CAD build for the part. Positions are in the model's coordinates, mm. A direction names the side the tool comes from. Round coordinates to 2 decimals unless told otherwise and drop trailing zeros. Order: outer loops, then holes, each group sorted by start corner. A loop starts at its lowest first (then second) coordinate and runs counter-clockwise, first axis right, second up.
Autodesk Inventor part; units mm, degrees
ref_plane "YZ Plane" through (0, 0, 0) normal (1, 0, 0) x (0, 1, 0)
ref_plane "XZ Plane" through (0, 0, 0) normal (0, 1, 0) x (-1, 0, 0)
ref_plane "XY Plane" through (0, 0, 0) normal (0, 0, 1) x (1, 0, 0)
sketch "Sketch1" plane through (0, 0, 0) normal (0, 1, 0) x (-1, 0, 0)
  line L0 (0, 0) -> (170, 0)
  line L1 (170, 0) -> (170, -132.9)
  line L2 (0, -132.9) -> (0, 0)
  line L3 (170, -132.9) -> (95, -132.9)
  line L4 (75, -132.9) -> (0, -132.9)
  line L5 (95, -132.9) -> (95, -127.9)
  line L6 (95, -127.9) -> (75, -127.9)
  line L7 (75, -127.9) -> (75, -132.9)
  dimension "d0" = 132.9
  dimension "d22" = 170
  dimension "d23" = 75
  dimension "d24" = 75
  dimension "d41" = 5
  dimension "d42" = 5
  dimension "d43" = 75
  dimension "d44" = 20
extrude "Extrusion1" add sketch "Sketch1" along normal blind 4.7625
sketch "Sketch2" plane through (0, 4.7625, 0) normal (0, 1, 0) x (1, 0, 0)
  line L0 (-170, 0) -> (0, 0)
  line L1 (0, 132.9) -> (-170, 132.9)
  line L2 (-170, 0) -> (-170, 132.9)
  line L3 (-170, 132.9) -> (-165.2375, 132.9)
  line L4 (-165.2375, 132.9) -> (-165.2375, 0)
  line L5 (-170, 0) -> (-165.2375, 0)
  line L6 (0, 0) -> (-4.7625, 0)
  line L7 (-4.7625, 0) -> (-4.7625, 132.9)
  line L8 (-4.7625, 132.9) -> (0, 132.9)
  line L9 (0, 0) -> (0, 132.9)
  line L10 (0, 132.9) -> (0, 0)
  dimension "d4" = 4.7625
  dimension "d5" = 4.7625
extrude "Extrusion2" add sketch "Sketch2" along normal blind 85.2375 contours L7 L1 L9 L0
sketch "Sketch3" plane through (0, 4.7625, 0) normal (0, 1, 0) x (1, 0, 0)
  point P0 (0, 0)
sketch "Sketch4" plane through (-170, 0, -132.9) normal (-1, 0, 0) x (0, 0, 1)
  line L0 (132.9, 4.7625) -> (217.7528, 89.6153)
  line L1 (0, 4.7625) -> (132.9, 4.7625)
  line L2 (132.9, 0) -> (132.9, 4.7625)
  line L3 (0, 0) -> (132.9, 0)
  line L4 (132.9, 0) -> (220.1341, 87.2341)
  line L5 (220.1341, 87.2341) -> (217.7528, 89.6153)
  line L6 (132.9, 4.7625) -> (132.9, 0)
  dimension "d8" = 120
  dimension "d9" = 45
sketch "Sketch5" plane through (0, 0, 0) normal (1, 0, 0) x (0, 0, -1)
  line L0 (0, 0) -> (0, 90)
  line L1 (0, 90) -> (-90, 90)
  line L2 (132.9, 0) -> (0, 0)
  line L3 (-90, 90) -> (0, 0)
  line L4 (0, 0) -> (0, 90)
  dimension "d11" = 45
extrude "Extrusion3" add sketch "Sketch5" against normal blind 105.2375
sketch "Sketch6" plane through (-105.2375, 0, 0) normal (-1, 0, 0) x (0, 0, 1)
  line L0 (0, 0) -> (0, 4.7625)
  line L1 (0, 4.7625) -> (0, 90)
  line L2 (-132.9, 90) -> (90, 90)
  line L3 (0, 90) -> (85.2375, 90)
  line L4 (85.2375, 90) -> (0, 4.7625)
  line L5 (0, 0) -> (90, 90)
extrude "Extrusion4" cut sketch "Sketch6" against normal blind 100.475 contours L1 L2 L4
sketch "Sketch7" plane through (-105.2375, 0, 0) normal (-1, 0, 0) x (0, 0, 1)
  line L0 (0, 4.7625) -> (0, 0)
  line L1 (0, 0) -> (90, 90)
  line L2 (85.2375, 90) -> (0, 4.7625)
  line L3 (90, 90) -> (85.2375, 90)
  line L4 (85.2375, 90) -> (0, 4.7625)
extrude "Extrusion5" add sketch "Sketch7" along normal blind 64.75
extrude "Extrusion6" add sketch "Sketch2" along normal blind 85.2375 contours L2 L1 L4 L0
sketch "Sketch8" plane through (-170, 0, -132.9) normal (-1, 0, 0) x (0, 0, 1)
  line L0 (0, 90) -> (222.9, 90)
  line L1 (132.9, 90) -> (218.1375, 90)
  line L2 (218.1375, 90) -> (132.9, 4.7625)
  line L3 (218.1375, 90) -> (132.9, 4.7625)
  line L4 (132.9, 4.7625) -> (132.9, 90)
  point P0 (132.9, 0)
extrude "Extrusion7" add sketch "Sketch8" against normal blind 4.7625
sketch "Sketch9" plane through (0, 0, -132.9) normal (1, 0, 0) x (0, 0, -1)
  line L0 (0, 0) -> (0, 90)
  line L1 (-5, 55) -> (0, 55)
  line L2 (0, 55) -> (0, 35)
  line L3 (0, 35) -> (-5, 35)
  line L4 (-5, 35) -> (-5, 55)
  line L5 (0, 90) -> (-222.9, 90)
  line L6 (0, 0) -> (-132.9, 0)
  dimension "d28" = 5
  dimension "d29" = 20
  dimension "d30" = 35
  dimension "d31" = 35
extrude "Extrusion8" cut sketch "Sketch9" against normal blind 4.7625
sketch "Sketch10" plane through (-170, 0, -132.9) normal (-1, 0, 0) x (0, 0, 1)
  line L0 (0, 0) -> (0, 90)
  line L1 (0, 55) -> (5, 55)
  line L2 (5, 55) -> (5, 35)
  line L3 (5, 35) -> (0, 35)
  line L4 (0, 35) -> (0, 55)
  line L5 (0, 90) -> (218.1375, 90)
  line L6 (132.9, 0) -> (0, 0)
  dimension "d34" = 20
  dimension "d35" = 5
  dimension "d36" = 35
  dimension "d37" = 35
extrude "Extrusion9" cut sketch "Sketch10" against normal blind 4.7625
fillet "Fillet1" radius 1 4 edges at (-167.6188, 55, -127.9) (-167.6188, 35, -127.9) (-2.3813, 35, -127.9) (-2.3813, 55, -127.9)
properties part number "OpticalDeviceMirrorPart"
1. Tool access for faces 5 (the face through (-75, 2, -130)), 6 (the face through (-84, 4.762, -66)), 7 (the face through (-168, 45, -127.9)): list every direction of +Z, -Z, +X, -X, +Y, -Y with a clear straight run to the whole face (end or side of a thin tool).
2. Pin check, flat tips, straight feed: P1, Ø1.4, axis at x = -86, y = 2, coming from the -Z side; P2, Ø6, axis at x = -29.5, y = 15, coming from the -Z side; P3, Ø1.5, axis at x = -61.5, y = 15, coming from the -Z side. Stop position of each tip, or through.
3. Cut at D-D, the plane z = -89. Write the cut outline in (x, y), and give its area (3 significant figures).
4. Cut at C-C, the plane x = -39. Write the cut outline in (y, z), and give its area (3 significant figures).
5. Drill centre lines: line 1 (X direction, y = 48, z = -94); line 2 (Y direction, x = -43, z = -54.5); line 3 (Z direction, x = -29, y = 34.5). Where is each one in solid material? Low to high.
6. Mould opens along X. For faces 1 (the face through (-83.88, 47.98, 43.22)), 2 (the face through (-2, 45, -127.9)), 3 (the face through (-4.762, 47, -47)), 4 (the face through (-170, 46, -50)) say: released by +X, released by -X, zero draft, split by the parting line, or undercut.
Outcome:
1. face 5: -Z, +Y, -Y
1. face 6: -Z, +Y
1. face 7: -Z, +X, -X
2. P1: stops at z = -127.9
2. P2: stops at z = 7.24
2. P3: stops at z = 9.49
3. outline: (-170, 0) - (0, 0) - (0, 90) - (-4.76, 90) - (-4.76, 4.76) - (-165.24, 4.76) - (-165.24, 90) - (-170, 90) - close
3. area: 1,620 mm2
4. outline: (0, -132.9) - (4.76, -132.9) - (4.76, 0) - (90, 85.24) - (90, 90) - (0, 0) - close
4. area: 1,050 mm2
5. line 1: x = -170 to -165.24, -4.76 to 0
5. line 2: y = 0 to 4.76
5. line 3: z = 29.74 to 34.5
6. face 1: undercut
6. face 2: zero draft
6. face 3: undercut
6. face 4: released by -X
